Can you work these out from the model? Positions are in its coordinate system, mm. A direction names the side the tool comes from. Round coordinates to 2 decimals unless told otherwise and drop trailing zeros. Loops run counter-clockwise (first coordinate to the right, second up) from the corner with the lowest first, then second, coordinate; pieces in that order, holes last. Notation, with made-up numbers: (77, 49.25) -> (96, 49.25) arc R8 ccw to (96, 59.25) -> close; hole circle Ø6 at (42, 17). An arc over 180 degrees is marked (long way). Write item = value, one per line.
Autodesk Inventor part; units mm, degrees
ref_plane "YZ Plane" through (0, 0, 0) normal (1, 0, 0) x (0, 1, 0)
ref_plane "XZ Plane" through (0, 0, 0) normal (0, 1, 0) x (-1, 0, 0)
ref_plane "XY Plane" through (0, 0, 0) normal (0, 0, 1) x (1, 0, 0)
sketch "Sketch1" plane through (0, 0, 0) normal (0, 0, 1) x (-1, 0, 0)
  line L0 (-57.15, 78.74) -> (57.15, 78.74)
  line L1 (57.15, 78.74) -> (57.15, -78.74)
  line L2 (57.15, -78.74) -> (-57.15, -78.74)
  line L3 (-57.15, -78.74) -> (-57.15, 78.74)
  line L4 (-57.15, 78.74) -> (57.15, -78.74) construction
  line L5 (57.15, 78.74) -> (-57.15, -78.74) construction
  point P0 (0, 0)
  dimension "d0" = 114.3
  dimension "d1" = 157.48
extrude "Extrusion1" add sketch "Sketch1" along normal blind 6.35
sketch "Sketch2" plane through (0, 0, 0) normal (0, 0, 1) x (1, 0, 0)
  line L0 (0, 106.68) -> (0, -106.68)
  line L1 (72.898, -1.6229) -> (-72.898, -1.6229)
  line L2 (0, -106.68) -> (0, 106.68)
  line L3 (-102.0572, 0) -> (102.0572, 0)
  point P0 (45.72, 45.72)
  point P1 (-46.228, 45.72)
  point P2 (45.72, -46.228)
  point P3 (-46.228, -46.228)
  point P4 (-45.72, 69.85)
  point P5 (-45.72, -69.85)
  point P6 (46.228, 69.85)
  point P7 (46.228, -69.85)
  dimension "d18" = 91.948
  dimension "d21" = 91.948
  dimension "d25" = 45.72
  dimension "d28" = 139.7
  dimension "d31" = 91.948
  dimension "d34" = 69.85
hole "Hole1" at (45.72, 45.72, 0) at (-46.228, 45.72, 0) at (-46.228, -46.228, 0) at (45.72, -46.228, 0) at (-45.72, 69.85, 0) at (46.228, 69.85, 0) at (-45.72, -69.85, 0) at (46.228, -69.85, 0) direction (0, 0, 1) diameter 7.62 end through all
sketch "Sketch6" plane through (0, 0, 6.35) normal (0, 0, 1) x (1, 0, 0)
  line L0 (-10.16, 10.16) -> (-43.434, 10.16)
  line L1 (-43.434, 10.16) -> (-43.434, 37.846)
  line L2 (-43.434, 37.846) -> (-10.16, 37.846)
  line L3 (-10.16, 37.846) -> (-10.16, 10.16)
  line L4 (-80.01, 0) -> (80.01, 0)
  line L5 (0, -110.236) -> (0, 110.236)
  line L6 (-43.434, 37.846) -> (-11.5677, 37.846) construction
  line L7 (-43.434, 37.846) -> (-7.62, 37.846) construction
  line L8 (-43.434, 37.846) -> (-34.4537, 46.8263)
  line L9 (-43.434, 37.846) -> (-30.734, 37.846) construction
  line L10 (-34.4537, 46.8263) -> (-10.16, 46.8263)
  line L11 (-10.16, 46.8263) -> (-10.16, 64.6111)
  line L12 (-10.16, 64.6111) -> (-34.4537, 64.6111)
  line L13 (-34.4537, 64.6111) -> (-34.4537, 46.8263)
  line L14 (-10.16, 46.8263) -> (-10.16, 37.846)
  line L15 (10.16, 10.16) -> (43.434, 10.16)
  line L16 (43.434, 10.16) -> (43.434, 37.846)
  line L17 (43.434, 37.846) -> (10.16, 37.846)
  line L18 (10.16, 37.846) -> (10.16, 10.16)
  line L19 (43.434, 37.846) -> (11.5677, 37.846) construction
  line L20 (43.434, 37.846) -> (7.62, 37.846) construction
  line L21 (43.434, 37.846) -> (34.4537, 46.8263)
  line L22 (43.434, 37.846) -> (30.734, 37.846) construction
  line L23 (34.4537, 46.8263) -> (10.16, 46.8263)
  line L24 (10.16, 46.8263) -> (10.16, 64.6111)
  line L25 (10.16, 64.6111) -> (34.4537, 64.6111)
  line L26 (34.4537, 64.6111) -> (34.4537, 46.8263)
  line L27 (10.16, 46.8263) -> (10.16, 37.846)
  line L28 (-10.16, -10.16) -> (-43.434, -10.16)
  line L29 (-43.434, -10.16) -> (-43.434, -37.846)
  line L30 (-43.434, -37.846) -> (-10.16, -37.846)
  line L31 (-10.16, -37.846) -> (-10.16, -10.16)
  line L32 (-43.434, -37.846) -> (-11.5677, -37.846) construction
  line L33 (-43.434, -37.846) -> (-7.62, -37.846) construction
  line L34 (-43.434, -37.846) -> (-34.4537, -46.8263)
  line L35 (-43.434, -37.846) -> (-30.734, -37.846) construction
  line L36 (-34.4537, -46.8263) -> (-10.16, -46.8263)
  line L37 (-10.16, -46.8263) -> (-10.16, -64.6111)
  line L38 (-10.16, -64.6111) -> (-34.4537, -64.6111)
  line L39 (-34.4537, -64.6111) -> (-34.4537, -46.8263)
  line L40 (-10.16, -46.8263) -> (-10.16, -37.846)
  line L41 (10.16, -10.16) -> (43.434, -10.16)
  line L42 (43.434, -10.16) -> (43.434, -37.846)
  line L43 (10.16, -37.846) -> (10.16, -10.16)
  line L44 (43.434, -37.846) -> (10.16, -37.846)
  line L45 (43.434, -37.846) -> (11.5677, -37.846) construction
  line L46 (43.434, -37.846) -> (30.734, -37.846) construction
  line L47 (10.16, -46.8263) -> (10.16, -37.846)
  line L48 (34.4537, -46.8263) -> (10.16, -46.8263)
  line L49 (43.434, -37.846) -> (34.4537, -46.8263)
  line L50 (10.16, -46.8263) -> (10.16, -64.6111)
  line L51 (10.16, -64.6111) -> (34.4537, -64.6111)
  line L52 (34.4537, -64.6111) -> (34.4537, -46.8263)
  line L53 (43.434, -37.846) -> (7.62, -37.846) construction
  point P0 (0, 0)
  dimension "d41" = 10.16
  dimension "d42" = 10.16
  dimension "d43" = 43.434
  dimension "d44" = 37.846
  dimension "d54" = 12.7
  dimension "d55" = 45
extrude "Extrusion3" cut sketch "Sketch6" against normal blind 25.4
equation "\"d12\" = d18"
properties part number "MotorAdapter"
1. We'd pull the mould along X, two halves only. Please class faces 3 (the flat face through (-22, -64.611, 3)), 4 (the flat face through (1, -1, 6.35)): released by +X, released by -X, zero draft, split by the parting line, or undercut.
Entries:
face_3 = undercut
face_4 = zero draft
2. For faces 1 (the flat face through (1, -78.74, 3)), 2 (the flat face through (39.01, -42.27, 3.22)), which set-ups out of +Z, -Z, +X, -X, +Y, -Y let a thin tool reach every point of the face, with its end or its side?
Entries:
face_1 = +Z, -Z, +X, -X, -Y
face_2 = +Z, -Z
3. I'm going to push a flat-ended pin straight in: pin 1 (6 mm diameter, centred on x = 45.72, y = -46.228, fed in from +Z). Where does the tip first touch, or does it pass through?
Entries:
pin_1 = through
4. Suppose I cut it at A-A, the plane y = 69.85. List the corners of the cut face in (x, z) for me, and give its area (3 significant figures).
Entries:
outline = (-57.15, 0) -> (-49.53, 0) -> (-49.53, 6.35) -> (-57.15, 6.35) -> close; (-41.91, 0) -> (42.42, 0) -> (42.42, 6.35) -> (-41.91, 6.35) -> close; (50.04, 0) -> (57.15, 0) -> (57.15, 6.35) -> (50.04, 6.35) -> close
area = 629 mm²
5. Suppose I cut it at C-C, the plane z = 2.25. Count the separate pieces of the cut face and the enclosed holes in it, and give its area (3 significant figures).
Entries:
separate_pieces = 1
enclosed_holes = 12
area = 11,200 mm²
6. Suppose I cut it at B-B, the plane x = -37.5. List the corners of the cut face in (y, z) for me, and give its area (3 significant figures).
Entries:
outline = (-78.74, 0) -> (-43.78, 0) -> (-43.78, 6.35) -> (-78.74, 6.35) -> close; (-10.16, 0) -> (10.16, 0) -> (10.16, 6.35) -> (-10.16, 6.35) -> close; (43.78, 0) -> (78.74, 0) -> (78.74, 6.35) -> (43.78, 6.35) -> close
area = 573 mm²
7. I need wall thicknesses on line 1 (Y direction, x = 34, z = 0.5); line 2 (X direction, y = 25, z = 2.25); line 3 (Y direction, x = 45.72, z = 4.5). Which ranges of each line are inside material? Lowest first, please. Write a range as [from, to].
Entries:
line_1 = [-78.74, -64.61], [-10.16, 10.16], [64.61, 78.74]
line_2 = [-57.15, -43.43], [-10.16, 10.16], [43.43, 57.15]
line_3 = [-78.74, -73.63], [-66.07, -50.04], [-42.42, 41.91], [49.53, 66.07], [73.63, 78.74]
